Geometry check sheet. Reference: the model listing, model coordinates, mm. A direction names the side the tool comes from. Give positions to 0.01 mm unless a question says otherwise; leave off trailing zeros. Write each loop counter-clockwise with the first axis right and the second up, starting at its lowest first coordinate (ties: lowest second). Pieces come first, ordered by that corner, then holes. Notation, with made-up numbers: (50.25, -37.5) -> (78.25, -37.5) arc R20 cw to (78.25, -18.5) -> close; hole circle Ø8 at (-24, 11.5). An arc over 180 degrees is marked (long way). One line per item, written item: value.
from build123d import *

# Parameters (mm, degrees)
SKETCH1_W           = 38.1
SKETCH1_H           = 38.1
BOSS_EXTRUDE1_DEPTH = 304.8
SKETCH2_R           = 5
CUT_EXTRUDE1_DEPTH  = 308.762168728
SKETCH4_R           = 2.5
CUT_EXTRUDE3_DEPTH  = 308.762168728
CIRPATTERN2_COUNT   = 6
SKETCH5_R           = 2.25
CUT_EXTRUDE4_DEPTH  = 308.762168728
CIRPATTERN3_COUNT   = 4
SKETCH6_W           = 88.9
SKETCH6_H           = 38.1
CUT_EXTRUDE5_DEPTH  = 28.575
SKETCH7_W           = 38.1
SKETCH7_H           = 6.35
CUT_EXTRUDE6_DEPTH  = 306.9883086


with BuildPart() as part:
    # Sketch1 → Boss-Extrude1 (new body)
    with BuildSketch(Plane.XY):
        Rectangle(SKETCH1_W, SKETCH1_H)
    extrude(amount=BOSS_EXTRUDE1_DEPTH)

    # Sketch2 → Cut-Extrude1 (cut, through all)
    with BuildSketch(Plane(origin=(19.05, 0, 0), x_dir=(0, 0, -1), z_dir=(1, 0, 0))):
        with Locations(Location((-19.05, -2, 0), (0, 0, 90))):
            Circle(SKETCH2_R)
        with Locations(Location((-64.05, 0, 0), (0, 0, 90))):
            Circle(SKETCH2_R)
    extrude(amount=-CUT_EXTRUDE1_DEPTH, mode=Mode.SUBTRACT)

    # Sketch4 → Cut-Extrude3 (cut, through all)
    with BuildSketch(Plane(origin=(19.05, 0, 0), x_dir=(0, 0, -1), z_dir=(1, 0, 0))):
        with Locations(Location((-78.768873451, 8.497872059, 0), (0, 0, 90))):
            Circle(SKETCH4_R)
    cut_extrude3 = extrude(amount=-CUT_EXTRUDE3_DEPTH, mode=Mode.SUBTRACT)

    # CirPattern2: Cut-Extrude3 ×6 about axis, 2 skipped
    cirpattern2_axis = Axis((0, 0, 64.05), (1, 0, 0))
    add([cut_extrude3.rotate(cirpattern2_axis, i * 360 / CIRPATTERN2_COUNT) for i in range(1, CIRPATTERN2_COUNT) if i not in (2, 5)], mode=Mode.SUBTRACT)

    # Sketch5 → Cut-Extrude4 (cut, through all)
    with BuildSketch(Plane(origin=(19.05, 0, 0), x_dir=(0, 0, -1), z_dir=(1, 0, 0))):
        with Locations(Location((-29.303048327, 8.253048327, 0), (0, 0, 90))):
            Circle(SKETCH5_R)
    cut_extrude4 = extrude(amount=-CUT_EXTRUDE4_DEPTH, mode=Mode.SUBTRACT)

    # CirPattern3: Cut-Extrude4 ×4 about axis
    cirpattern3_axis = Axis((0, -2, 19.05), (1, 0, 0))
    for i in range(1, CIRPATTERN3_COUNT):
        add(cut_extrude4.rotate(cirpattern3_axis, i * 360 / CIRPATTERN3_COUNT), mode=Mode.SUBTRACT)

    # Sketch6 → Cut-Extrude5 (cut)
    with BuildSketch(Plane(origin=(19.05, 0, 0), x_dir=(0, 0, -1), z_dir=(1, 0, 0))):
        with Locations((-44.45, 0)):
            Rectangle(SKETCH6_W, SKETCH6_H)
    extrude(amount=-CUT_EXTRUDE5_DEPTH, mode=Mode.SUBTRACT)

    # Sketch7 → Cut-Extrude6 (cut, through all)
    with BuildSketch(Plane.XY.offset(304.8)):
        with Locations((0, 15.875)):
            Rectangle(SKETCH7_W, SKETCH7_H)
    extrude(amount=-CUT_EXTRUDE6_DEPTH, mode=Mode.SUBTRACT)


solid = part.part
1) Mould release check, pull along Z, two halves, no side actions. Record for faces 1 (the flat face through (0, -3, 304.8)), 2 (the flat face through (0, 12.7, 188)), 3 (the cylindrical face through (-14.221, -7.956, 51.772)): released by +Z, released by -Z, zero draft, split by the parting line, or undercut.
Verdict:
face 1: released by +Z
face 2: zero draft
face 3: undercut
2) Scan lines: probe 1 along Z at (x, y) = (0, -5); probe 2 along Z at (x, y) = (-12.5, 10); probe 3 along Z at (x, y) = (-15, 0). Record each from-to range of solid material in increasing order.
Verdict:
probe 1: 88.9 to 304.8
probe 2: 0 to 7.38, 10.21 to 27.89, 30.72 to 47.33, 51.33 to 76.77, 80.77 to 304.8
probe 3: 0 to 14.47, 23.63 to 59.05, 69.05 to 304.8
3) Tool access check on faces 4 (the flat face through (0, -19.05, 184)), 5 (the flat face through (-9.525, -3, 45)). Record the directions out of +Z, -Z, +X, -X, +Y, -Y that give a thin tool (end or side, any length) a straight path to the whole face; none if there is none.
Verdict:
face 4: +Z, -Z, +X, -X, -Y
face 5: -Z, +X, +Y, -Y
4) Sectioned sample at C-C on x = 3.5. Record the cut outline in (y, z), plus the area to 3 significant figures.
Verdict:
outline: (-19.05, 88.9) -> (12.7, 88.9) -> (12.7, 304.8) -> (-19.05, 304.8) -> close
area: 6,850 mm^2
5) Depth check by flat-ended pin: pin 1 Ø8 at (x, y) = (-1, -2) entering from -Z; pin 2 Ø4.5 at (y, z) = (8.5, 49.33) entering from +X; pin 3 Ø16 at (y, z) = (-2, 19.05) entering from +X (3 decimals). Enter the tip coordinate at first touch or a pass-through.
Verdict:
pin 1: z = 88.9
pin 2: through
pin 3: x = -9.525
6) Sectioned sample at B-B on y = -2. Record the cut outline in (x, z) (3 decimals), plus the area to 3 significant figures.
Verdict:
outline: (-19.05, 0) -> (-9.525, 0) -> (-9.525, 14.05) -> (-19.05, 14.05) -> close; (-19.05, 24.05) -> (-9.525, 24.05) -> (-9.525, 59.467) -> (-19.05, 59.467) -> close; (-19.05, 68.633) -> (-9.525, 68.633) -> (-9.525, 88.9) -> (19.05, 88.9) -> (19.05, 304.8) -> (-19.05, 304.8) -> close
area: 8,890 mm^2
7) Sectioned sample at A-A on z = 64.05. Record the cut outline in (x, y) (3 decimals), plus the area to 3 significant figures.
Verdict:
outline: (-19.05, -19.05) -> (-9.525, -19.05) -> (-9.525, -5) -> (-19.05, -5) -> close; (-19.05, 5) -> (-9.525, 5) -> (-9.525, 12.7) -> (-19.05, 12.7) -> close
area: 207 mm^2
